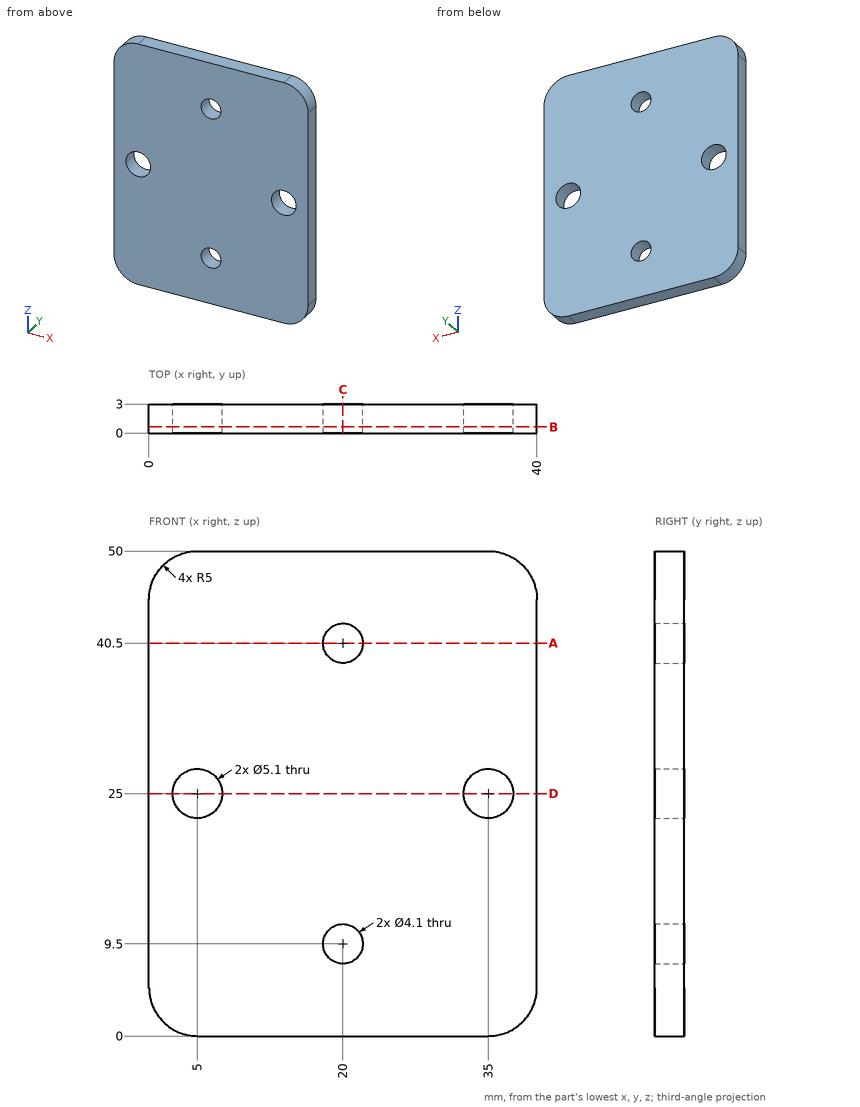
Print and shaded views of the part. All mm, measured from the part's lowest x, y and z. Round coordinates to 2 decimals unless told otherwise and drop trailing zeros. Order: outer loops, then holes, each group sorted by start corner. A loop starts at its lowest first (then second) coordinate and runs counter-clockwise, first axis right, second up.
Q1. Slice it at D-D (z = 25). Write the cut outline in (x, y).
Q2. Drop a flat-ended pin along its axis: pin 1 (4 mm diameter, centred on x = 36, z = 36, fed in from -Y). Give the stop position or say it passes through.
Q3. Slice it at B-B (y = 0.65). Write the cut outline in (x, z), and give its area (3 significant figures).
Q4. Slice it at C-C (x = 20). Write the cut outline in (y, z).
Q5. Wall check: L1, parallel to Z at x = 20, y = 1.55; L2, parallel to Z at x = 35, y = 1.8; L3, parallel to Z at x = 4, y = 2.75. Give the ranges that are in metal, low to high.
Q6. Slice it at A-A (z = 40.5). Write the cut outline in (x, y).
Results below:
1. outline: (0, 0) - (2.45, 0) - (2.45, 3) - (0, 3) - close; (7.55, 0) - (32.45, 0) - (32.45, 3) - (7.55, 3) - close; (37.55, 0) - (40, 0) - (40, 3) - (37.55, 3) - close
2. pin 1: stops at y = 0
3. outline: (0, 5) arc R5 ccw to (5, 0) - (35, 0) arc R5 ccw to (40, 5) - (40, 45) arc R5 ccw to (35, 50) - (5, 50) arc R5 ccw to (0, 45) - close; hole circle Ø5.1 at (5, 25); hole circle Ø4.1 at (20, 9.5); hole circle Ø4.1 at (20, 40.5); hole circle Ø5.1 at (35, 25)
3. area: 1,910 mm2
4. outline: (0, 0) - (3, 0) - (3, 7.45) - (0, 7.45) - close; (0, 11.55) - (3, 11.55) - (3, 38.45) - (0, 38.45) - close; (0, 42.55) - (3, 42.55) - (3, 50) - (0, 50) - close
5. L1: z = 0 to 7.45, 11.55 to 38.45, 42.55 to 50
5. L2: z = 0 to 22.45, 27.55 to 50
5. L3: z = 0.1 to 22.65, 27.35 to 49.9
6. outline: (0, 0) - (17.95, 0) - (17.95, 3) - (0, 3) - close; (22.05, 0) - (40, 0) - (40, 3) - (22.05, 3) - close
